Answer from the drawing. Dimensions are ordinates in mm from the lowest x, y and z of the part. A direction names the side the tool comes from. Round coordinates to 2 decimals unless told otherwise and drop trailing zeros. Loops run counter-clockwise (first coordinate to the right, second up) from the corner with the lowest first, then second, coordinate; pieces in that order, holes last. Notation, with made-up numbers: (-31, -13) -> (-9, -13) arc R25 ccw to (-9, 7) -> close; hole circle Ø11 at (54, 54.5). An arc over 180 degrees is marked (long way). One line per question, with ' | ' between items.
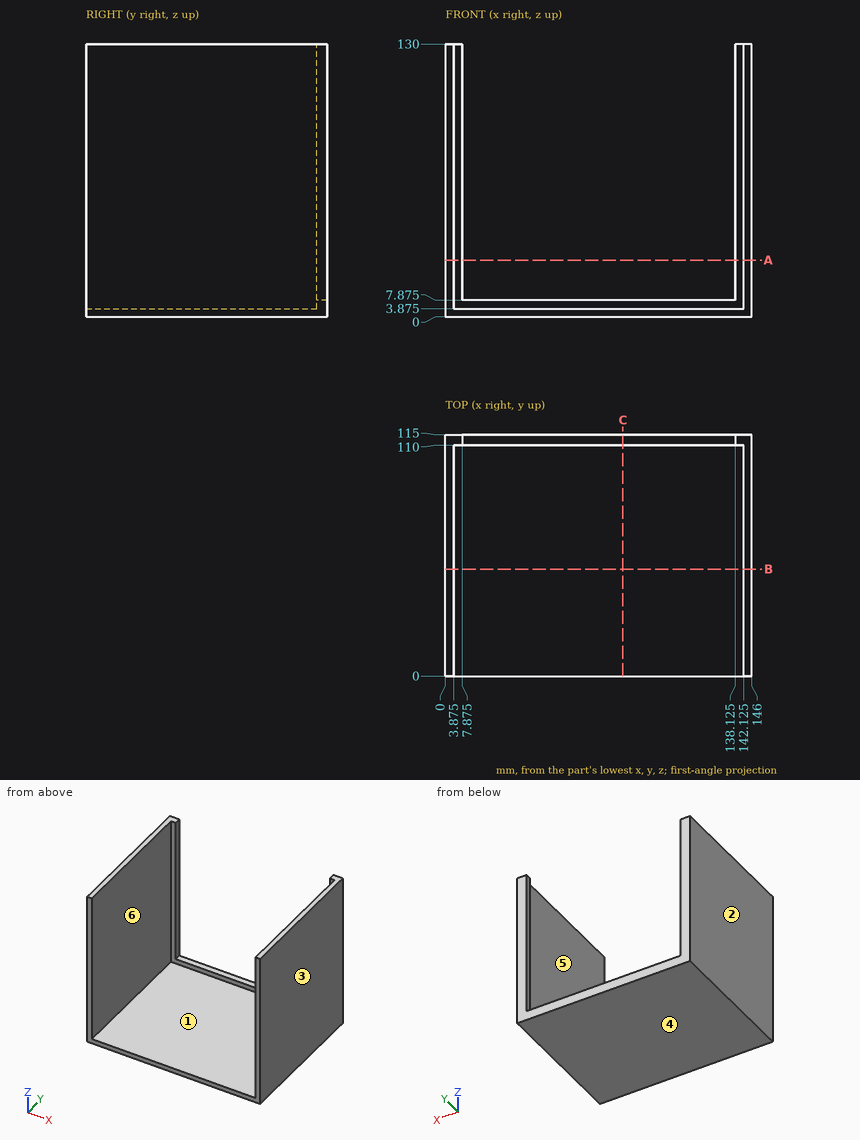
Q1. For a pull along X with two mould halves and no side action, classify the marked faces 3, 4, 5 and 6 as pulls with the +X half, pulls with the -X half, needs draft (parallel to the pull), parting line crosses it, or undercut.
Numbers:
face 3: pulls with the +X half | face 4: needs draft | face 5: undercut | face 6: undercut
Q2. A cutting plane is placed at A-A on z = 27. Give the vertices of the cut face in (x, y) (3 decimals), plus the area to 3 significant figures.
Numbers:
outline: (0, 0) -> (3.875, 0) -> (3.875, 110) -> (7.875, 110) -> (7.875, 115) -> (0, 115) -> close; (138.125, 110) -> (142.125, 110) -> (142.125, 0) -> (146, 0) -> (146, 115) -> (138.125, 115) -> close | area: 931 mm^2
Q3. Given pin 1 Ø10 at (x, y) = (86.5, 77) entering from +Z (3 decimals); pin 2 Ø2.5 at (x, y) = (74, 113) entering from +Z (3 decimals), each flat-ended and moving along its own axis, determine where each tip first touches the part or whether it passes through.
Numbers:
pin 1: z = 3.875 | pin 2: z = 7.875
Q4. Find the intervals of material crossed by line 1 (X direction, y = 66, z = 41.5) (3 decimals); line 2 (Z direction, x = 14, y = 71) (3 decimals), in increasing order. Write a range as from..to.
Numbers:
line 1: 0..3.875, 142.125..146 | line 2: 0..3.875
Q5. A cutting plane is placed at C-C on x = 84.5. Give the vertices of the cut face in (y, z) (3 decimals), plus the area to 3 significant figures.
Numbers:
outline: (0, 0) -> (115, 0) -> (115, 7.875) -> (110, 7.875) -> (110, 3.875) -> (0, 3.875) -> close | area: 466 mm^2
Q6. A cutting plane is placed at B-B on y = 51. Give the vertices of the cut face in (x, z) (3 decimals), plus the area to 3 significant figures.
Numbers:
outline: (0, 0) -> (146, 0) -> (146, 130) -> (142.125, 130) -> (142.125, 3.875) -> (3.875, 3.875) -> (3.875, 130) -> (0, 130) -> close | area: 1,540 mm^2
Q7. For the marked faces 1 and 2, determine the directions among +Z, -Z, +X, -X, +Y, -Y from which every point of the face is accessible in a straight line to the end or side of a thin tool.
Numbers:
face 1: +Z, -Y | face 2: +Z, -Z, -X, +Y, -Y
